```python
from build123d import *

# Parameters (mm, degrees)
SKETCH1_R               = 5
BOSS_EXTRUDE1_DEPTH     = 5
SKETCH2_R               = 3
BOSS_EXTRUDE2_DEPTH     = 13
SKETCH3_R               = 1.9
CUT_EXTRUDE1_DEPTH      = 10
CUT_EXTRUDE5_DEPTH      = 20.339079606
CUT_EXTRUDE5_DEPTH_BACK = 0.4
SKETCH7_R               = 1.8


with BuildPart() as part:
    # Sketch1 → Boss-Extrude1 (new body)
    with BuildSketch(Plane(origin=(0, 0, 0), x_dir=(1, 0, 0), z_dir=(0, 1, 0))):
        with Locations(Location((0, 0, 0), (0, 0, 270))):
            Circle(SKETCH1_R)
    extrude(amount=BOSS_EXTRUDE1_DEPTH)

    # Sketch2 → Boss-Extrude2 (add)
    with BuildSketch(Plane(origin=(0, 5, 0), x_dir=(1, 0, 0), z_dir=(0, 1, 0))):
        with Locations(Location((0, 0, 0), (0, 0, 90))):
            Circle(SKETCH2_R)
    extrude(amount=BOSS_EXTRUDE2_DEPTH)

    # Sketch3 → Cut-Extrude1 (cut)
    with BuildSketch(Plane.XZ):
        with Locations(Location((0, 0, 0), (0, 0, 270))):
            Circle(SKETCH3_R)
    extrude(amount=-CUT_EXTRUDE1_DEPTH, mode=Mode.SUBTRACT)

    # Sketch7 → Cut-Extrude5 (cut, two sides: drawn at the far end of the back side and taken through both)
    with BuildSketch(Plane.XY.offset(-CUT_EXTRUDE5_DEPTH_BACK)):
        with Locations((0, 13.5)):
            Circle(SKETCH7_R)
    extrude(amount=CUT_EXTRUDE5_DEPTH + CUT_EXTRUDE5_DEPTH_BACK, mode=Mode.SUBTRACT)


solid = part.part
```
For this review, take the finished solid that the model builds, in its own axes (mm). A direction names the side the tool comes from. Give positions to 0.01 mm unless a question says otherwise; leave off trailing zeros. Write each loop counter-clockwise with the first axis right and the second up, starting at its lowest first coordinate (ties: lowest second). Pieces come first, ordered by that corner, then holes. Notation, with made-up numbers: M 3.5,48 L 20.5,48 A17 ccw 20.5,75 Z; hole C 35.25,-17.5 d6. An arc over 180 degrees is marked long. One line per item, written item: value.
1) Take a section at D-D, the plane z = -1. Write out the cut boundary in (x, y).
Results are:
outline: M -4.9,0 L -1.62,0 L -1.62,10 L 1.62,10 L 1.62,0 L 4.9,0 L 4.9,5 L 2.83,5 L 2.83,18 L -2.83,18 L -2.83,5 L -4.9,5 Z
2) For P1, Ø1.5, axis at x = -3, z = -0.5, coming from the -Y side; P2, Ø1.5, axis at x = 3.5, y = 13.5, coming from the -Z side; P3, Ø3, axis at x = 0, y = 13.5, coming from the -Z side; P4, Ø1.1, axis at x = 0.5, z = -0.5, coming from the -Y side, all flat-tipped, find the tip position at first contact; note any pin that passes through.
Results are:
P1: stops at y = 0
P2: stops at z = -1.2
P3: stops at z = -3
P4: stops at y = 10
3) Take a section at A-A, the plane z = 0. Write out the cut boundary in (x, y).
Results are:
outline: M -5,0 L -1.9,0 L -1.9,10 L 1.9,10 L 1.9,0 L 5,0 L 5,5 L 3,5 L 3,18 L -3,18 L -3,5 L -5,5 Z; hole C 0,13.5 d3.6
4) For faces 1 (the cylindrical face through (1.717, 14.041, 1.276)), 2 (the flat face through (-3.3, 5, -0.1)), 3 (the cylindrical face through (-4.88, 2.46, -1.08)), 4 (the cylindrical face through (-0.728, 4.93, -1.755)), list the 3-axis set-ups (+Z, -Z, +X, -X, +Y, -Y) from which the entire face can be reached by the end or side of a thin tool; tool diameter is ignored.
Results are:
face 1: +Z
face 2: +Y
face 3: +Y, -Y
face 4: -Y
5) For line 1 (Y direction, x = 0, z = 1); line 2 (Y direction, x = -3.5, z = 3.25); line 3 (X direction, y = 2.25, z = -1), list the stretches that pass through material, from the lowest coordinate up. Write a range as from..to.
Results are:
line 1: y = 10..11.7, 15.3..18
line 2: y = 0..5
line 3: x = -4.9..-1.62, 1.62..4.9
6) The part is to be moulded in two halves that separate along X. For faces 5 (the cylindrical face through (-0.9, 11.41, -2.86)), 6 (the flat face through (0.1, 0, 2.2)), 7 (the flat face through (0, 10, 0)), say which applies: +X half, -X half, draft (parallel to the pull), parting line (faces both ways), or undercut.
Results are:
face 5: parting line
face 6: draft
face 7: undercut
7) Take a section at B-B, the plane x = 0. Write out the cut boundary in (y, z).
Results are:
outline: M 0,-5 L 5,-5 L 5,-3 L 18,-3 L 18,3 L 15.3,3 L 15.3,-0.4 L 11.7,-0.4 L 11.7,3 L 5,3 L 5,5 L 0,5 L 0,1.9 L 10,1.9 L 10,-1.9 L 0,-1.9 Z
8) Take a section at C-C, the plane y = 9.75. Write out the cut boundary in (x, z).
Results are:
outline: C 0,0 d6; hole C 0,0 d3.8
